Verification items for the finished model (mm, model axes). A direction names the side the tool comes from. Give positions to 0.01 mm unless a question says otherwise; leave off trailing zeros. Order: outer loops, then holes, each group sorted by start corner. A loop starts at its lowest first (then second) coordinate and runs counter-clockwise, first axis right, second up. Notation, with made-up numbers: (89.5, 17) - (134.5, 17) arc R18 ccw to (134.5, 43) - close; hole circle Ø5 at (35.5, 83.5). An arc over 180 degrees is marked (long way). Answer as a JSON object with one key per item and string values.
```python
from build123d import *

# Parameters (mm, degrees)
F0_W           = 20
F0_H           = 130
F1_DEPTH       = 6
F3_D           = 4
F3_DEPTH       = 20
F3_CBORE_D     = 7.3
F3_CBORE_DEPTH = 3.6
F5_D           = 7
F5_DEPTH       = 20
F7_D           = 6
F7_DEPTH       = 20
F8_SIZE        = 2
F9_SIZE        = 0.5


with BuildPart() as f1:
    # F0 (on Top) → F1 (new body)
    with BuildSketch(Plane.XY):
        Rectangle(F0_W, F0_H)
    extrude(amount=F1_DEPTH)

    # F3
    with Locations(Plane.XY.offset(6)):
        with Locations((0, 34.5), (0, -34.5)):
            CounterBoreHole(F3_D / 2, F3_CBORE_D / 2, F3_CBORE_DEPTH, depth=F3_DEPTH)

    # F5
    with Locations(Plane.XY.offset(6)):
        with Locations((-10, 44.5), (-10, -44.5)):
            Hole(F5_D / 2, depth=F5_DEPTH)

    # F7
    with Locations(Plane(origin=(0, 0, 0), x_dir=(1, 0, 0), z_dir=(0, 0, -1))):
        with Locations((0, -57.5), (0, 57.5)):
            Hole(F7_D / 2, depth=F7_DEPTH)

    # F8
    f8_edges = [f1.edges().sort_by_distance(p)[0] for p in [
        (-10, -65, 3),
        (10, -65, 3),
        (-10, 65, 3),
        (10, 65, 3),
    ]]
    chamfer(f8_edges, length=F8_SIZE)

    # F9
    f9_edges = [f1.edges().sort_by_distance(p)[0] for p in [
        (-10, -55.5, 0),
        (-9, -64, 0),
        (-6.5, -44.5, 0),
        (0, -65, 0),
        (-10, 0, 0),
        (9, -64, 0),
        (-6.5, 44.5, 0),
        (10, 0, 0),
        (-10, 55.5, 0),
        (9, 64, 0),
        (-9, 64, 0),
        (0, 65, 0),
        (-3, -57.5, 0),
        (-2, -34.5, 0),
        (-2, 34.5, 0),
        (-3, 57.5, 0),
        (-10, -55.5, 6),
        (-9, -64, 6),
        (-6.5, -44.5, 6),
        (0, -65, 6),
        (-10, 0, 6),
        (9, -64, 6),
        (-6.5, 44.5, 6),
        (10, 0, 6),
        (-10, 55.5, 6),
        (9, 64, 6),
        (-9, 64, 6),
        (0, 65, 6),
        (-3, -57.5, 6),
        (-3.65, -34.5, 6),
        (-3.65, 34.5, 6),
        (-3, 57.5, 6),
    ]]
    chamfer(f9_edges, length=F9_SIZE)


solid = f1.part
```
(1) Section check B-B (z = 4.25). Record the cut outline in (x, y), then the cut area to 3 significant figures.
Computed values:
{"outline": "(-10, -63) - (-8, -65) - (8, -65) - (10, -63) - (10, 63) - (8, 65) - (-8, 65) - (-10, 63) - (-10, 48) arc R3.5 cw to (-10, 41) - (-10, -41) arc R3.5 cw to (-10, -48) - close; hole circle Ø7.3 at (0, -34.5); hole circle Ø7.3 at (0, 34.5); hole circle Ø6 at (0, -57.5); hole circle Ø6 at (0, 57.5)", "area": "2,410 mm²"}
(2) Section check C-C (y = 57.5). Record the cut outline in (x, z).
Computed values:
{"outline": "(-10, 0.5) - (-9.5, 0) - (-3.5, 0) - (-3, 0.5) - (-3, 5.5) - (-3.5, 6) - (-9.5, 6) - (-10, 5.5) - close; (3, 0.5) - (3.5, 0) - (9.5, 0) - (10, 0.5) - (10, 5.5) - (9.5, 6) - (3.5, 6) - (3, 5.5) - close"}
(3) Section check D-D (x = 0). Count the separate pieces of the cut face and the enclosed holes in it, then the cut area to 3 significant figures.
Computed values:
{"separate pieces": "5", "enclosed holes": "0", "area": "634 mm²"}
(4) Material ranges on line 1 along Y through (x, z) = (0, 3.35); line 2 along Y through (x, z) = (1, 4.75); line 3 along X through (y, z) = (57.5, 2.7), recorded low to high. Write a range as [from, to].
Computed values:
{"line 1": "y = [-65, -60.5], [-54.5, -38.15], [-30.85, 30.85], [38.15, 54.5], [60.5, 65]", "line 2": "y = [-65, -60.33], [-54.67, -38.01], [-30.99, 30.99], [38.01, 54.67], [60.33, 65]", "line 3": "x = [-10, -3], [3, 10]"}
(5) Gauge pin test, flat ends, axial feed: pin 1 Ø3.5 at (x, y) = (1, 34) entering from +Z; pin 2 Ø6 at (x, y) = (-1, -34.5) entering from +Z. Record the tip position at first contact, or that the pin passes through.
Computed values:
{"pin 1": "stops at z = 2.4", "pin 2": "stops at z = 5.85"}
(6) Release check for a two-part mould opening along Y. For faces 3 (the cylindrical face through (-0.791, -38.063, 3.972)), 4 (the flat face through (-9, -64, 3)), 5 (the cylindrical face through (0.391, 54.526, 3.035)), 6 (the flat face through (-8.81, 63.84, 5.75)) record: pulls with the +Y half, pulls with the -Y half, needs draft (parallel to the pull), parting line crosses it, or undercut.
Computed values:
{"face 3": "undercut", "face 4": "pulls with the -Y half", "face 5": "undercut", "face 6": "pulls with the +Y half"}
(7) Section check A-A (y = 34.5). Record the cut outline in (x, z).
Computed values:
{"outline": "(-10, 0.5) - (-9.5, 0) - (-2.5, 0) - (-2, 0.5) - (-2, 2.4) - (-3.65, 2.4) - (-3.65, 5.5) - (-4.15, 6) - (-9.5, 6) - (-10, 5.5) - close; (2, 0.5) - (2.5, 0) - (9.5, 0) - (10, 0.5) - (10, 5.5) - (9.5, 6) - (4.15, 6) - (3.65, 5.5) - (3.65, 2.4) - (2, 2.4) - close"}
(8) Access from +Z, -Z, +X, -X, +Y, -Y to the whole of each face (thin tool, end or side, straight path). Record for faces 1 (the conical face through (-6.365, 44.58, 0.365)), 2 (the flat face through (2, -36, 2.4)).
Computed values:
{"face 1": "-Z, -X", "face 2": "+Z"}
